from build123d import *

# Parameters (mm, degrees)
F0_W     = 139.7
F0_H     = 88.9
F1_DEPTH = 1219.2
F2_W     = 88.9
F2_H     = 88.9
F3_DEPTH = 38.1
F4_R     = 4.7625
F5_DEPTH = 25.4


with BuildPart() as f1:
    # F0 (on Top) → F1 (new body, symmetric)
    with BuildSketch(Plane.XY):
        Rectangle(F0_W, F0_H)
    extrude(amount=F1_DEPTH, both=True)

    # F2 (on face) → F3 (cut)
    with BuildSketch(Plane.YZ.offset(69.85)):
        with Locations((0, 1022.35)):
            Rectangle(F2_W, F2_H)
        with Locations((0, 273.05)):
            Rectangle(F2_W, F2_H)
    extrude(amount=-F3_DEPTH, mode=Mode.SUBTRACT)

    # F4 (on face) → F5 (cut)
    with BuildSketch(Plane(origin=(-69.85, 0, 0), x_dir=(0, -1, 0), z_dir=(-1, 0, 0))):
        with Locations((0, -558.8)):
            Circle(F4_R)
        with Locations((0, 1143)):
            Circle(F4_R)
        with Locations((0, 431.8)):
            Circle(F4_R)
    extrude(amount=-F5_DEPTH, mode=Mode.SUBTRACT)


solid = f1.part
Could you check a few things on this model? Use its own coordinates, in mm. A direction names the side the tool comes from. Give positions to 0.01 mm unless a question says otherwise; leave off trailing zeros. Order: outer loops, then holes, each group sorted by start corner. A loop starts at its lowest first (then second) coordinate and runs counter-clockwise, first axis right, second up.
Item 1: I need wall thicknesses on line 1 (Z direction, x = -59.5, y = 0); line 2 (Z direction, x = 37.5, y = -2.5); line 3 (Y direction, x = -52, z = 431.8). Which ranges of each line are inside material? Lowest first, please.
Item 2: I'm going to push flat-ended pins straight in: pin 1 (3 mm diameter, centred on y = 0, z = -559, fed in from -X); pin 2 (7.5 mm diameter, centred on y = 2, z = 1144.5, fed in from -X). Where does each tip first touch, or does it pass through?
Item 3: For faces 1 (the face through (-69.85, -1, 17)), 2 (the face through (51, -1, 317.5)), which set-ups out of +Z, -Z, +X, -X, +Y, -Y let a thin tool reach every point of the face, with its end or its side?
Item 4: If we section it at A-A, the plane y = -23: Write out the boundary of the cut face in (x, z).
Item 5: If we mould it in two halves opening along Z, with no side actions, what happens to faces 3 (the face through (-1, 1, -1219.2)), 4 (the face through (-1, 44.45, 17)), 5 (the face through (51, -1, 1066.8)), 6 (the face through (31.75, -1, 1023))? For each: pulls with the +Z half, pulls with the -Z half, needs draft (parallel to the pull), parting line crosses it, or undercut.
Values:
1. line 1: z = -1219.2 to -563.56, -554.04 to 427.04, 436.56 to 1138.24, 1147.76 to 1219.2
1. line 2: z = -1219.2 to 228.6, 317.5 to 977.9, 1066.8 to 1219.2
1. line 3: y = -44.45 to -4.76, 4.76 to 44.45
2. pin 1: stops at x = -44.45
2. pin 2: stops at x = -69.85
3. face 1: +Z, -Z, -X, +Y, -Y
3. face 2: +X, +Y, -Y
4. outline: (-69.85, -1219.2) - (69.85, -1219.2) - (69.85, 228.6) - (31.75, 228.6) - (31.75, 317.5) - (69.85, 317.5) - (69.85, 977.9) - (31.75, 977.9) - (31.75, 1066.8) - (69.85, 1066.8) - (69.85, 1219.2) - (-69.85, 1219.2) - close
5. face 3: pulls with the -Z half
5. face 4: needs draft
5. face 5: undercut
5. face 6: undercut
